Source: three-view drawing plus pictorial views. Frame: mm from the lowest corner of the part. Coordinates: 2 decimals unless noted, no trailing zeros. Write each loop counter-clockwise with the first axis right and the second up, starting at its lowest first coordinate (ties: lowest second). Pieces come first, ordered by that corner, then holes. Notation, with made-up numbers: (-6.5, -32.5) - (32.5, -32.5) arc R9 ccw to (32.5, -24.5) - close; hole circle Ø6 at (61.25, 66.25). An arc over 180 degrees is marked (long way). Put each result on its own line as item: value. Start each with the question number.
1. Cut plane D-D, the plane x = 77. Return loops of the section in (y, z).
2. Cut plane A-A, the plane x = 41. Return loops of the section in (y, z), and give its area (3 significant figures).
3. Line query: line 1 (Y direction, x = 6, z = 4.5); line 2 (X direction, y = 5.5, z = 0.5); line 3 (Y direction, x = 42.5, z = 6). Output: solid intervals per line, ascending.
4. Cut plane B-B, the plane z = 1.5. Count the separate pieces of the cut face and the enclosed holes in it, and give its area (3 significant figures).
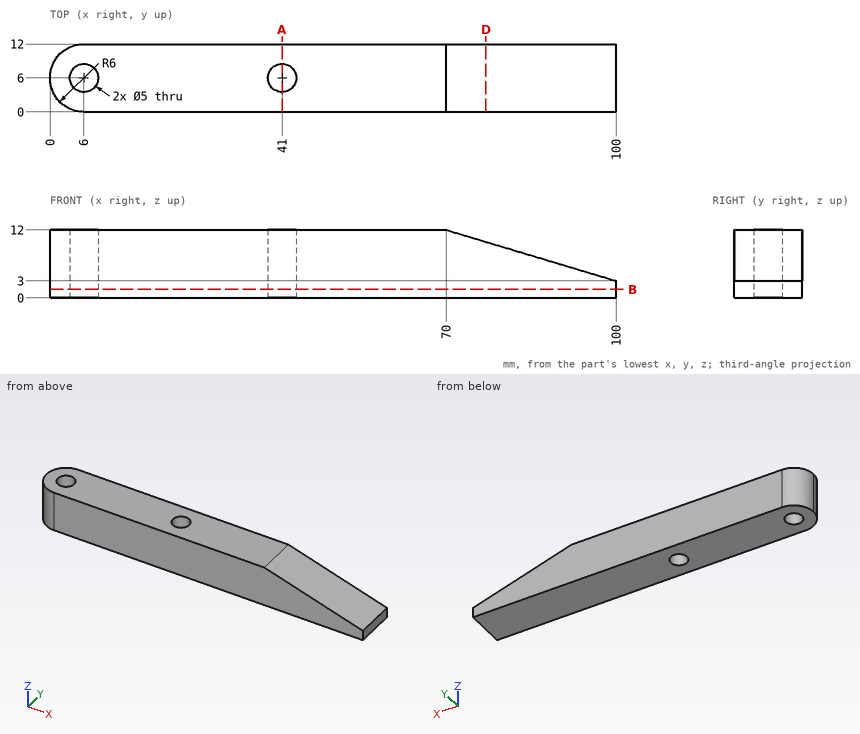
Report:
1. outline: (0, 0) - (12, 0) - (12, 9.9) - (0, 9.9) - close
2. outline: (0, 0) - (3.5, 0) - (3.5, 12) - (0, 12) - close; (8.5, 0) - (12, 0) - (12, 12) - (8.5, 12) - close
2. area: 84.0 mm^2
3. line 1: y = 0 to 3.5, 8.5 to 12
3. line 2: x = 0.02 to 3.55, 8.45 to 38.55, 43.45 to 100
3. line 3: y = 0 to 4, 8 to 12
4. separate pieces: 1
4. enclosed holes: 2
4. area: 1,150 mm^2
